```python
from build123d import *

# Parameters (mm, degrees)
SKETCH1_R           = 2.1
BOSS_EXTRUDE1_DEPTH = 3


with BuildPart() as part:
    # Sketch1 → Boss-Extrude1 (new body)
    with BuildSketch(Plane(origin=(0, 0, 0), x_dir=(1, 0, 0), z_dir=(0, 1, 0))):
        with BuildLine():
            ThreePointArc((-6.773431823, -3.22034491), (0, -7.5), (6.773431823, -3.22034491))
            ThreePointArc((6.773431823, -3.22034491), (12.3053133, 3.157859017), (20.332742003, 5.773883946))
            ThreePointArc((20.332742003, 5.773883946), (27.062266479, 15.791255027), (15.507209772, 19.271899728))
            ThreePointArc((15.507209772, 19.271899728), (0, 14.113175247), (-15.507209772, 19.271899728))
            ThreePointArc((-15.507209772, 19.271899728), (-27.062266479, 15.791255027), (-20.332742003, 5.773883946))
            ThreePointArc((-20.332742003, 5.773883946), (-12.3053133, 3.157859017), (-6.773431823, -3.22034491))
        make_face()
        with Locations(Location((0, 0, 0), (0, 0, 270))):
            Circle(SKETCH1_R, mode=Mode.SUBTRACT)
        with Locations(Location((20, 13.266499161, 0), (0, 0, 270))):
            Circle(SKETCH1_R, mode=Mode.SUBTRACT)
        with Locations(Location((-20, 13.266499161, 0), (0, 0, 270))):
            Circle(SKETCH1_R, mode=Mode.SUBTRACT)
    extrude(amount=BOSS_EXTRUDE1_DEPTH)


solid = part.part
```
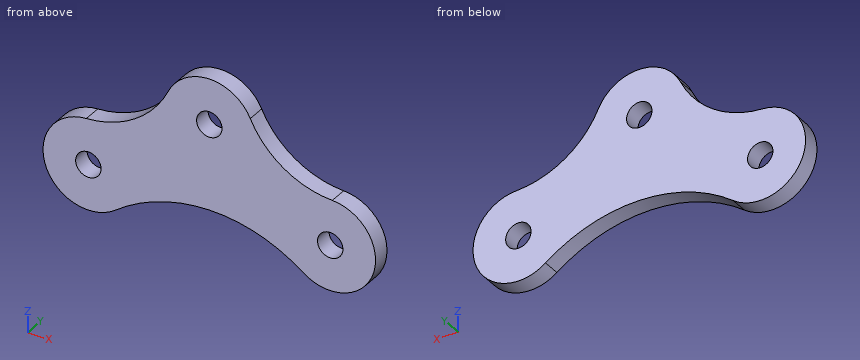
Verification items for the finished model (mm, model axes). Coordinates: 2 decimals unless noted, no trailing zeros. Loops run counter-clockwise (first coordinate to the right, second up) from the corner with the lowest first, then second, coordinate; pieces in that order, holes last. Notation, with made-up numbers: (-7, -37.75) - (-3, -37.75) arc R26 ccw to (-3, -6.75) - close; hole circle Ø8 at (56, 48.5). An arc over 180 degrees is marked (long way). Return JSON: item names as keys, results as strings.
1. Thickness scan on L1, parallel to X at y = 0.3, z = -13; L2, parallel to X at y = 0.5, z = -11.75; L3, parallel to Z at x = 1, y = 0.9. Record the ranges inside material, lowest first.
Established:
{"L1": "x = -27.5 to -22.08, -17.92 to 17.92, 22.08 to 27.5", "L2": "x = -27.35 to -21.45, -18.55 to 18.55, 21.45 to 27.35", "L3": "z = -14.13 to -1.85, 1.85 to 7.43"}
2. Section check A-A, the plane y = 1.7. Record the boundary of the cut face in (x, z), then the cut area to 3 significant figures.
Established:
{"outline": "(-20.33, -5.77) arc R7.5 ccw (long way) to (-15.51, -19.27) arc R25.89 cw to (15.51, -19.27) arc R7.5 ccw (long way) to (20.33, -5.77) arc R15.79 cw to (6.77, 3.22) arc R7.5 ccw to (-6.77, 3.22) arc R15.79 cw to start; hole circle Ø4.2 at (-20, -13.27); hole circle Ø4.2 at (0, 0); hole circle Ø4.2 at (20, -13.27)", "area": "811 mm2"}
3. Section check D-D, the plane z = -6.75. Record the boundary of the cut face in (x, y).
Established:
{"outline": "(-23.71, 0) - (23.71, 0) - (23.71, 3) - (-23.71, 3) - close"}
4. Section check C-C, the plane z = 0. Record the boundary of the cut face in (x, y).
Established:
{"outline": "(-8.81, 0) - (-2.1, 0) - (-2.1, 3) - (-8.81, 3) - close; (2.1, 0) - (8.81, 0) - (8.81, 3) - (2.1, 3) - close"}
5. Go/stop test with a flat-tipped pin: pin 1 (2 mm diameter, centred on x = 18.5, z = -3, fed in from -Y). Record where the tip stops, or that it passes through.
Established:
{"pin 1": "passes through"}
6. Section check B-B, the plane x = 0. Record the boundary of the cut face in (y, z), then the cut area to 3 significant figures.
Established:
{"outline": "(0, -14.11) - (3, -14.11) - (3, -2.1) - (0, -2.1) - close; (0, 2.1) - (3, 2.1) - (3, 7.5) - (0, 7.5) - close", "area": "52.2 mm2"}
